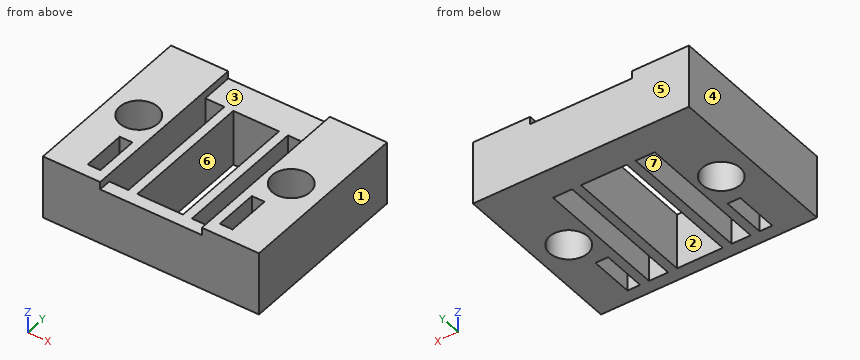
Autodesk Inventor part; units mm, degrees
ref_plane "YZ Plane" through (0, 0, 0) normal (1, 0, 0) x (0, 1, 0)
ref_plane "XZ Plane" through (0, 0, 0) normal (0, 1, 0) x (-1, 0, 0)
ref_plane "XY Plane" through (0, 0, 0) normal (0, 0, 1) x (1, 0, 0)
sketch "スケッチ1" plane through (0, 0, 0) normal (0, 0, 1) x (1, 0, 0)
  line L0 (8.5, 7) -> (-8.5, 7)
  line L1 (-8.5, 7) -> (-8.5, -7)
  line L2 (-8.5, -7) -> (8.5, -7)
  line L3 (8.5, -7) -> (8.5, 7)
  line L4 (8.5, 7) -> (-8.5, -7) construction
  line L5 (-8.5, 7) -> (8.5, -7) construction
  circle A0 centre (-6, 0) radius 1.5
  circle A1 centre (6, 0) radius 1.5
  line L6 (-8.5, -6) -> (8.5, -6)
  line L7 (-8.5, 4.5) -> (8.5, 4.5)
  line L8 (-4, -7) -> (-4, 7)
  line L9 (4, -7) -> (4, 7)
  line L10 (2.5, -6) -> (2.5, 4.5)
  line L11 (-2.5, -6) -> (-2.5, 4.5)
  line L12 (1.8, -6) -> (1.8, 4.5)
  line L13 (-1.8, -6) -> (-1.8, 4.5)
  point P0 (0, 0)
  point P1 (-4, -6)
  point P2 (-4, 4.5)
  point P3 (4, -6)
  point P4 (4, 4.5)
  dimension "d0" = 17
  dimension "d1" = 14
  dimension "d2" = 3
  dimension "d3" = 3
  dimension "d4" = 2.5
  dimension "d5" = 4.5
  dimension "d6" = 4.5
  dimension "d7" = 1.5
  dimension "d8" = 1.5
  dimension "d9" = 1
  dimension "d16" = 0.7
  dimension "d17" = 0.7
extrude "押し出し1" add sketch "スケッチ1" along normal blind 5 contours L3 L7 L9 L0 | L9 L7 L8 L0 | L3 L6 L9 L7 | L8 L7 L1 L0 | L3 L2 L9 L6 | L8 L6 L1 L7 | L10 L6 L12 L7 | L9 L2 L8 L6 | L7 L13 L6 L11 | L8 L2 L1 L6
sketch "スケッチ2" plane through (0, 0, 5) normal (0, 0, 1) x (1, 0, 0)
  line L0 (8.5, 7) -> (-8.5, 7)
  line L1 (0, 7) -> (-4, 7)
  line L2 (-4, 7) -> (-4, -7)
  line L3 (-8.5, -7) -> (8.5, -7)
  line L4 (-4, -7) -> (4, -7)
  line L5 (4, -7) -> (4, 7)
  line L6 (4, 7) -> (0, 7)
  point P0 (0, 0)
  dimension "d12" = 4
  dimension "d13" = 8
extrude "押し出し2" cut sketch "スケッチ2" against normal blind 0.6
sketch "スケッチ3" plane through (0, 0, 0) normal (0, 0, -1) x (-1, 0, 0)
  line L0 (4.7, -6) -> (4.7, -2.5)
  line L1 (4, -6) -> (4, 4.5)
  line L2 (4.7, -6) -> (5.7, -6)
  line L3 (5.7, -6) -> (5.7, -2.5)
  line L4 (5.7, -2.5) -> (4.7, -2.5)
  line L5 (-4.7, -6) -> (-4.7, -2.5)
  line L6 (-4.7, -2.5) -> (-5.7, -2.5)
  line L7 (-5.7, -2.5) -> (-5.7, -6)
  line L8 (-5.7, -6) -> (-4.7, -6)
  line L9 (8.5, -7) -> (-8.5, -7)
  point P0 (0, 0)
  point P1 (5.2, -6)
  dimension "d18" = 3.5
  dimension "d19" = 0.7
  dimension "d20" = 1
  dimension "d21" = 1
  dimension "d24" = 1
  dimension "d25" = 1
  dimension "d26" = 3.5
extrude "押し出し3" cut sketch "スケッチ3" against normal blind 10
properties part number "greiper_TPU" material "ゴム、シリコーン"
Input: part model. Units: mm. Frame: model coordinates. Face numbers are marked on the shaded views. A direction names the side the tool comes from. Coordinates: 2 decimals unless noted, no trailing zeros. Order: outer loops, then holes, each group sorted by start corner. A loop starts at its lowest first (then second) coordinate and runs counter-clockwise, first axis right, second up. Notation, with made-up numbers: M 81,-34 L 103,-34 A16 ccw 103,-13 Z; hole C 62.5,-31 d3. An arc over 180 degrees is marked long. Write item = value, one per line. Start each with the question number.
(1) Section D-D on y = -1.75. Output: boundary loops of the cut face in (x, z), and give its area (3 significant figures).
(2) Pull-direction query (X, two-part tool) for the marked faces 4, 5, 6 and 7; classes: released by +X, released by -X, zero draft, split by the parting line, or undercut.
(3) Section B-B on y = 0. Output: boundary loops of the cut face in (x, z).
(4) Line query: line 1 along X through (y, z) = (-3.75, 1.95); line 2 along X through (y, z) = (3, 2.85); line 3 along Y through (x, z) = (-1, 2). Output: solid intervals per line, ascending. Write a range as [from, to].
(5) Section A-A on x = -6. Output: boundary loops of the cut face in (y, z), and give its area (3 significant figures).
(6) Reachability of the marked faces 1, 2 and 3 from +Z, -Z, +X, -X, +Y, -Y: full face, straight path, thin tool, end or side. Return the list, or none.
(7) Section C-C on z = 1.65. Output: boundary loops of the cut face in (x, y), and give its area (3 significant figures).
Result set:
q1.outline = M -8.5,0 L -4,0 L -4,5 L -8.5,5 Z; M -2.5,0 L -1.8,0 L -1.8,4.4 L -2.5,4.4 Z; M 1.8,0 L 2.5,0 L 2.5,4.4 L 1.8,4.4 Z; M 4,0 L 8.5,0 L 8.5,5 L 4,5 Z
q1.area = 51.2 mm²
q2.face_4 = released by -X
q2.face_5 = zero draft
q2.face_6 = undercut
q2.face_7 = undercut
q3.outline = M -8.5,0 L -7.5,0 L -7.5,5 L -8.5,5 Z; M -4.5,0 L -4,0 L -4,5 L -4.5,5 Z; M -2.5,0 L -1.8,0 L -1.8,4.4 L -2.5,4.4 Z; M 1.8,0 L 2.5,0 L 2.5,4.4 L 1.8,4.4 Z; M 4,0 L 4.5,0 L 4.5,5 L 4,5 Z; M 7.5,0 L 8.5,0 L 8.5,5 L 7.5,5 Z
q4.line_1 = [-8.5, -5.7], [-4.7, -4], [-2.5, -1.8], [1.8, 2.5], [4, 4.7], [5.7, 8.5]
q4.line_2 = [-8.5, -4], [-2.5, -1.8], [1.8, 2.5], [4, 8.5]
q4.line_3 = [-7, -6], [4.5, 7]
q5.outline = M -7,0 L -1.5,0 L -1.5,5 L -7,5 Z; M 1.5,0 L 7,0 L 7,5 L 1.5,5 Z
q5.area = 55.0 mm²
q6.face_1 = +Z, -Z, +X, +Y, -Y
q6.face_2 = +Z, -Z
q6.face_3 = +Z, +Y, -Y
q7.outline = M -8.5,-7 L 8.5,-7 L 8.5,7 L -8.5,7 Z; hole C -6,0 d3; hole M -5.7,-6 L -4.7,-6 L -4.7,-2.5 L -5.7,-2.5 Z; hole M -4,-6 L -2.5,-6 L -2.5,4.5 L -4,4.5 Z; hole M -1.8,-6 L 1.8,-6 L 1.8,4.5 L -1.8,4.5 Z; hole M 2.5,-6 L 4,-6 L 4,4.5 L 2.5,4.5 Z; hole C 6,0 d3; hole M 4.7,-6 L 5.7,-6 L 5.7,-2.5 L 4.7,-2.5 Z
q7.area = 148 mm²
